```python
from build123d import *

# Parameters (mm, degrees)
BOSS_EXTRUDE2_DEPTH      = 35
CUT_EXTRUDE8_DEPTH       = 1
CUT_EXTRUDE8_DEPTH_BACK  = 36
CUT_EXTRUDE10_DEPTH      = 1
CUT_EXTRUDE10_DEPTH_BACK = 70.282032303


with BuildPart() as part:
    # Sketch1 → Boss-Extrude2 (new body)
    with BuildSketch(Plane(origin=(0, 0, 0), x_dir=(1, 0, 0), z_dir=(0, 1, 0))):
        Polygon((0, 40), (-34.641016151, 20), (-34.641016151, -20), (0, -40), (34.641016151, -20), (34.641016151, 20), align=None)
    extrude(amount=BOSS_EXTRUDE2_DEPTH)

    # Sketch8 → Cut-Extrude8 (cut, two sides)
    with BuildSketch(Plane(origin=(0, 35, 0), x_dir=(1, 0, 0), z_dir=(0, 1, 0))) as cut_extrude8_sk:
        with BuildLine():
            Line((-6, 29.265974935), (6, 29.265974935))
            Line((6, 29.265974935), (6, 24.269322199))
            ThreePointArc((6, 24.269322199), (17.67766953, 17.67766953), (24.269322199, 6))
            Line((24.269322199, 6), (30.040393537, 6))
            Line((30.040393537, 6), (30.040393537, -6))
            Line((30.040393537, -6), (24.269322199, -6))
            ThreePointArc((24.269322199, -6), (17.67766953, -17.67766953), (6, -24.269322199))
            Line((6, -24.269322199), (6, -30.734025065))
            Line((6, -30.734025065), (-6, -30.734025065))
            Line((-6, -30.734025065), (-6, -24.269322199))
            ThreePointArc((-6, -24.269322199), (-17.67766953, -17.67766953), (-24.269322199, -6))
            Line((-24.269322199, -6), (-29.959606463, -6))
            Line((-29.959606463, -6), (-29.959606463, 6))
            Line((-29.959606463, 6), (-24.269322199, 6))
            ThreePointArc((-24.269322199, 6), (-17.67766953, 17.67766953), (-6, 24.269322199))
            Line((-6, 24.269322199), (-6, 29.265974935))
        make_face()
    extrude(amount=CUT_EXTRUDE8_DEPTH, mode=Mode.SUBTRACT)
    extrude(cut_extrude8_sk.sketch, amount=-CUT_EXTRUDE8_DEPTH_BACK, mode=Mode.SUBTRACT)

    # Sketch9 → Cut-Extrude10 (cut, two sides)
    with BuildSketch(Plane.ZY.offset(34.641016151)) as cut_extrude10_sk:
        Polygon((40, 35), (-40, 15), (-40, 35), (-20, 35), (20, 35), align=None)
    extrude(amount=CUT_EXTRUDE10_DEPTH, mode=Mode.SUBTRACT)
    extrude(cut_extrude10_sk.sketch, amount=-CUT_EXTRUDE10_DEPTH_BACK, mode=Mode.SUBTRACT)


solid = part.part
```
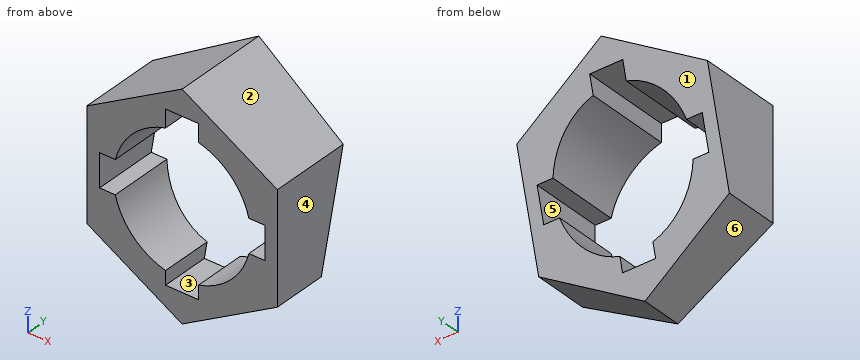
Can you work these out from the model? Positions are in its coordinate system, mm. Face numbers are marked on the shaded views. A direction names the side the tool comes from. Coordinates: 2 decimals unless noted, no trailing zeros. Order: outer loops, then holes, each group sorted by start corner. A loop starts at its lowest first (then second) coordinate and runs counter-clockwise, first axis right, second up.
1. I'm going to push flat-ended pins straight in: pin 1 (2 mm diameter, centred on x = 21, z = 30.5, fed in from -Y); pin 2 (6.5 mm diameter, centred on x = -26.5, y = 19, fed in from -Z); pin 3 (7 mm diameter, centred on y = 9, z = 28, fed in from -X); pin 4 (1.7 mm diameter, centred on x = 26, y = 19, fed in from -Z). Where does each tip first touch, or does it pass through?
2. Thinking about a two-plate mould opening in Z: for the marked faces 1, 2, 3 and 4, which applies, +Z half, -Z half, draft (parallel to the pull), parting line (faces both ways), or undercut?
3. For the marked faces 5 and 6, which set-ups out of +Z, -Z, +X, -X, +Y, -Y let a thin tool reach every point of the face, with its end or its side?
4. If we section it at A-A (y = 7.5): Please give me the cut outline in (x, z).
5. I need wall thicknesses on line 1 (Z direction, x = -27, y = 9.5); line 2 (X direction, y = 21, z = 19); line 3 (Z direction, x = 15.5, y = 13.5). Which ranges of each line are inside material? Lowest first, please.
6. If we section it at B-B (z = -1): Please give me the cut outline in (x, y).
7. If we section it at D-D (z = -34.5): Please give me the cut outline in (x, y) (3 decimals), then the cut area to 3 significant figures.
8. If we section it at C-C (x = 15): Please give me the cut outline in (y, z).
Entries:
1. pin 1: passes through
1. pin 2: stops at z = -26.54
1. pin 3: stops at x = -26.85
1. pin 4: stops at z = -25.43
2. face 1: -Z half
2. face 2: +Z half
2. face 3: undercut
2. face 4: draft
3. face 5: +Y, -Y
3. face 6: -Z, -X, +Y, -Y
4. outline: (-34.64, -20) - (0, -40) - (34.64, -20) - (34.64, 20) - (0, 40) - (-34.64, 20) - close; hole (-29.96, -6) - (-24.27, -6) arc R25 ccw to (-6, -24.27) - (-6, -29.27) - (6, -29.27) - (6, -24.27) arc R25 ccw to (24.27, -6) - (30.04, -6) - (30.04, 6) - (24.27, 6) arc R25 ccw to (6, 24.27) - (6, 30.73) - (-6, 30.73) - (-6, 24.27) arc R25 ccw to (-24.27, 6) - (-29.96, 6) - close
5. line 1: z = -24.41 to -6, 6 to 24.41
5. line 2: x = -34.64 to -16.25, 16.25 to 34.64
5. line 3: z = -31.05 to -19.62, 19.62 to 31.05
6. outline: (-34.64, 0) - (-29.96, 0) - (-29.96, 24.75) - (-34.64, 24.75) - close; (30.04, 0) - (34.64, 0) - (34.64, 24.75) - (30.04, 24.75) - close
7. outline: (-9.526, 0) - (9.526, 0) - (9.526, 16.375) - (-9.526, 16.375) - close
7. area: 312 mm2
8. outline: (0, -31.34) - (17.17, -31.34) - (20, -20) - (0, -20) - close; (0, 20) - (30, 20) - (32.83, 31.34) - (0, 31.34) - close
